Source: three-view drawing plus pictorial views. Frame: mm from the lowest corner of the part. A direction names the side the tool comes from. Coordinates: 2 decimals unless noted, no trailing zeros. Write each loop counter-clockwise with the first axis right and the second up, starting at its lowest first coordinate (ties: lowest second). Pieces come first, ordered by that corner, then holes. Notation, with made-up numbers: (62.5, 17.25) - (89.5, 17.25) arc R36 ccw to (89.5, 51.25) - close; hole circle Ø7 at (30.5, 30). An arc over 180 degrees is marked (long way). Put each result on its own line as item: value. Start each with the question number.
1. Pin query (flat end, axial travel): pin 1 (3 mm diameter, centred on x = 34, y = 25.5, fed in from +Z) (1 decimal); pin 2 (5.5 mm diameter, centred on y = 6, z = 46.5, fed in from -X); pin 3 (1 mm diameter, centred on x = 21, z = 7, fed in from -Y). Return the tip coordinate at first contact, or that it passes through.
2. Pull-direction query (X, two-part tool) for the marked faces 1, 2, 3 and 4; classes: released by +X, released by -X, zero draft, split by the parting line, or undercut.
3. Access query for the marked faces 5, 6 and 7. Directions: +Z, -Z, +X, -X, +Y, -Y. A direction counts if a zero-diameter tool reaches every point of the face in a straight line with its end or side. Return the directions, or none.
4. Line query: line 1 (X direction, y = 26, z = 31.5) (1 decimal); line 2 (X direction, y = 32, z = 40.5) (1 decimal); line 3 (Z direction, x = 42, y = 30). Output: solid intervals per line, ascending.
5. Cut plane D-D, the plane y = 10.5. Return loops of the section in (x, z) (1 decimal).
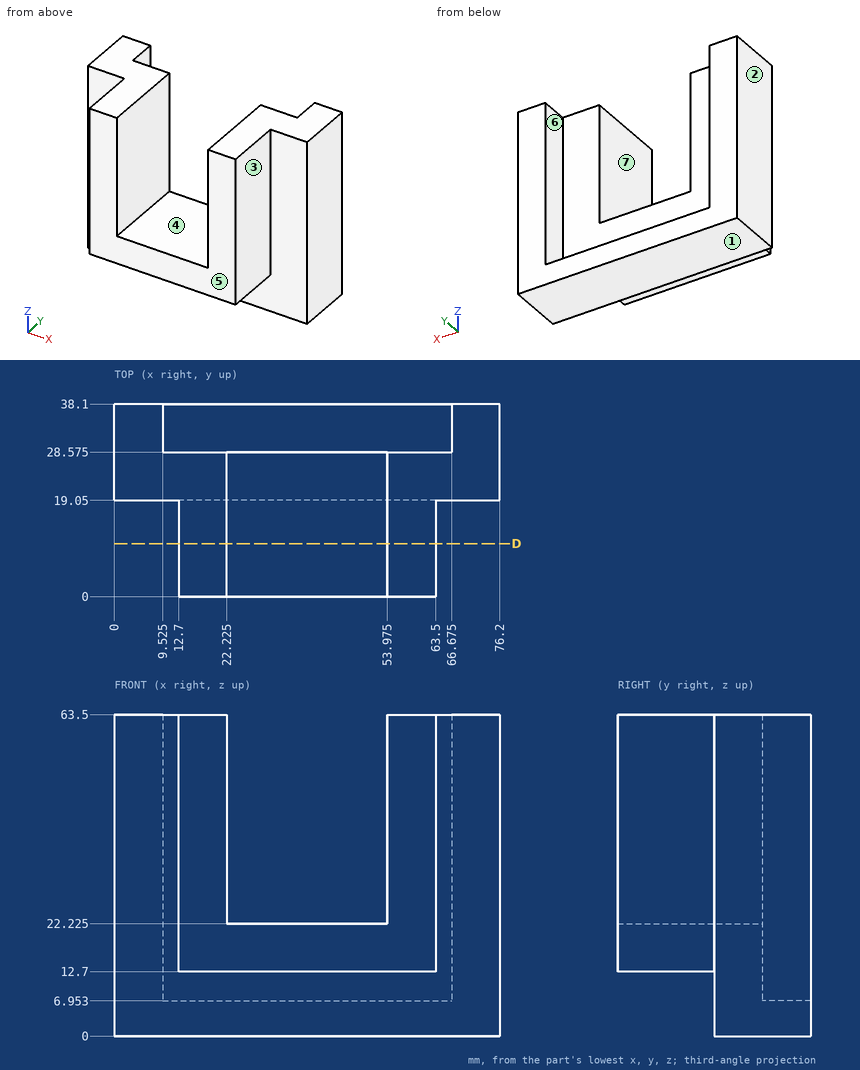
Report:
1. pin 1: stops at z = 22.2
1. pin 2: stops at x = 12.7
1. pin 3: stops at y = 19.05
2. face 1: zero draft
2. face 2: released by -X
2. face 3: released by +X
2. face 4: undercut
3. face 5: +Z, -Z, +X, -X, -Y
3. face 6: +Z, +Y
3. face 7: +Z, +Y, -Y
4. line 1: x = 0 to 22.2, 54 to 76.2
4. line 2: x = 0 to 9.5, 66.7 to 76.2
4. line 3: z = 0 to 6.95
5. outline: (12.7, 12.7) - (63.5, 12.7) - (63.5, 63.5) - (54, 63.5) - (54, 22.2) - (22.2, 22.2) - (22.2, 63.5) - (12.7, 63.5) - close
